```python
from build123d import *

# Parameters (mm, degrees)
SKETCH1_R           = 28.2
SKETCH1_R_2         = 3
BOSS_EXTRUDE1_DEPTH = 4
SKETCH1_5_R         = 6
BOSS_EXTRUDE3_DEPTH = 17
CHAMFER1_SIZE       = 6
CHAMFER1_SIZE2      = 4
FILLET3_R           = 3
CHAMFER3_SIZE       = 0.4
CHAMFER3_SIZE2      = 0.692820323


with BuildPart() as part:
    # Sketch1 → Boss-Extrude1 (new body)
    with BuildSketch(Plane.XY):
        Circle(SKETCH1_R)
        with Locations((-22.289967255, 8.342503208)):
            Circle(SKETCH1_R_2, mode=Mode.SUBTRACT)
        with Locations((-3.920163919, 23.474929496)):
            Circle(SKETCH1_R_2, mode=Mode.SUBTRACT)
        with Locations((18.369803336, 15.132426289)):
            Circle(SKETCH1_R_2, mode=Mode.SUBTRACT)
        with Locations((22.289967255, -8.342503208)):
            Circle(SKETCH1_R_2, mode=Mode.SUBTRACT)
        with Locations((3.920163919, -23.474929496)):
            Circle(SKETCH1_R_2, mode=Mode.SUBTRACT)
        with Locations((-18.369803336, -15.132426289)):
            Circle(SKETCH1_R_2, mode=Mode.SUBTRACT)
    extrude(amount=BOSS_EXTRUDE1_DEPTH)

    # Sketch1<5> → Boss-Extrude3 (add)
    with BuildSketch(Plane.XY):
        Circle(SKETCH1_5_R)
    extrude(amount=BOSS_EXTRUDE3_DEPTH)

    # Chamfer1
    chamfer1_edges = [part.edges().sort_by_distance(p)[0] for p in [
        (-6, 0, 4),
    ]]
    chamfer1_side = [part.faces().sort_by_distance(p)[0] for p in [
        (-6, 0, 10.5),
    ]]
    chamfer(chamfer1_edges, length=CHAMFER1_SIZE, length2=CHAMFER1_SIZE2, reference=chamfer1_side[0])

    # Fillet3
    fillet3_edges = [part.edges().sort_by_distance(p)[0] for p in [
        (-10, 0, 4),
    ]]
    fillet(fillet3_edges, radius=FILLET3_R)

    # Chamfer3
    chamfer3_edges = [part.edges().sort_by_distance(p)[0] for p in [
        (-6, 0, 17),
    ]]
    chamfer3_side = [part.faces().sort_by_distance(p)[0] for p in [
        (0, 0, 17),
    ]]
    chamfer(chamfer3_edges, length=CHAMFER3_SIZE, length2=CHAMFER3_SIZE2, reference=chamfer3_side[0])


solid = part.part
```
Geometry: final body of the model. Coordinates: model frame, mm. A direction names the side the tool comes from. Round coordinates to 2 decimals unless told otherwise and drop trailing zeros. Loops run counter-clockwise (first coordinate to the right, second up) from the corner with the lowest first, then second, coordinate; pieces in that order, holes last. Notation, with made-up numbers: (-39, 51) -> (-11, 51) arc R21 cw to (-11, 87) -> close; hole circle Ø3 at (10, 20.5). An arc over 180 degrees is marked (long way). Use one line per item in the form item = value.
Item 1: Draft query along Y for faces 1 (the conical face through (-1.343, 6.047, 9.708)), 2 (the cylindrical face through (-20.91, 5.68, 1.97)), 3 (the flat face through (0, 0, 17)), 4 (the cylindrical face through (19.983, 17.662, 1.972)). Return one class per face: released by +Y, released by -Y, zero draft, split by the parting line, or undercut.
Evaluation:
face_1 = split by the parting line
face_2 = undercut
face_3 = zero draft
face_4 = undercut
Item 2: Cut plane A-A on x = 16.5. Output: boundary loops of the cut face in (y, z), then the cut area to 3 significant figures.
Evaluation:
outline = (-22.87, 0) -> (12.79, 0) -> (12.79, 4) -> (-22.87, 4) -> close; (17.48, 0) -> (22.87, 0) -> (22.87, 4) -> (17.48, 4) -> close
area = 164 mm2
Item 3: Contact query for flat-ended pins moving along their axis: pin 1 Ø5.5 at (x, y) = (22.29, -8.34) entering from -Z; pin 2 Ø5 at (x, z) = (-1.5, 10) entering from -Y; pin 3 Ø8 at (x, z) = (17.5, 5) entering from -Y; pin 4 Ø4 at (y, z) = (-2.5, 3) entering from -X. Output: stop coordinate, or through.
Evaluation:
pin_1 = through
pin_2 = -7.57
pin_3 = -24.69
pin_4 = -28.2
Item 4: Material intervals for probe 1 along Z at (x, y) = (-10.5, 17); probe 2 along Y at (x, z) = (4, 2); probe 3 along Z at (x, y) = (-3.5, -6.5), sorted ascending.
Evaluation:
probe_1 = 0 to 4
probe_2 = -27.91 to -26.47, -20.48 to 27.91
probe_3 = 0 to 7.93
Item 5: Cut plane D-D on z = 2.25. Output: boundary loops of the cut face in (x, y), then the cut area to 3 significant figures.
Evaluation:
outline = circle Ø56.4 at (0, 0); hole circle Ø6 at (-22.29, 8.34); hole circle Ø6 at (-18.37, -15.13); hole circle Ø6 at (-3.92, 23.47); hole circle Ø6 at (3.92, -23.47); hole circle Ø6 at (18.37, 15.13); hole circle Ø6 at (22.29, -8.34)
area = 2,330 mm2
Item 6: Access query for faces 5 (the cylindrical face through (-6, 0, 13)), 6 (the cylindrical face through (3.53, -20.5, 1.97)). Directions: +Z, -Z, +X, -X, +Y, -Y. A direction counts if a zero-diameter tool reaches every point of the face in a straight line with its end or side. Return the directions, or none.
Evaluation:
face_5 = +Z
face_6 = +Z, -Z
Item 7: Cut plane B-B on y = 0. Output: boundary loops of the cut face in (x, z), then the cut area to 3 significant figures.
Evaluation:
outline = (-28.2, 0) -> (28.2, 0) -> (28.2, 4) -> (11.61, 4) arc R3 cw to (9.11, 5.34) -> (6, 10) -> (6, 16.31) -> (5.6, 17) -> (-5.6, 17) -> (-6, 16.31) -> (-6, 10) -> (-9.11, 5.34) arc R3 cw to (-11.61, 4) -> (-28.2, 4) -> close
area = 406 mm2
